```python
from build123d import *

# Parameters (mm, degrees)
F1_DEPTH = 63.5
F2_DEPTH = 25.4
F3_DEPTH = 7.9375
F0_W     = 21.7925966091
F0_H     = 28.575


with BuildPart() as f1:
    # F0 (on Front) → F1 (new body, symmetric)
    with BuildSketch(Plane.XZ):
        Polygon((31.6835418344, -20.7545107607), (-31.8164581656, -20.7545107607), (-31.8164581656, -39.8045107607), (50.7335418344, -39.8045107607), (50.7335418344, -20.7545107607), align=None)
    extrude(amount=F1_DEPTH, both=True)

    # F0 (on Front) → F2 (join, symmetric)
    with BuildSketch(Plane.XZ):
        with BuildLine():
            Line((31.6835418344, 16.0500892393), (31.6835418344, -20.7545107607))
            Line((31.6835418344, -20.7545107607), (50.7335418344, -20.7545107607))
            Line((50.7335418344, -20.7545107607), (50.7335418344, 16.0500892393))
            ThreePointArc((50.7335418344, 16.0500892393), (55.383221683, 27.2754093906), (66.6085418344, 31.9250892393))
            Line((66.6085418344, 31.9250892393), (77.2256346173, 31.9250892393))
            Line((77.2256346173, 31.9250892393), (77.2256346173, 50.9750892393))
            Line((77.2256346173, 50.9750892393), (66.6085418344, 50.9750892393))
            add(Edge.make_bspline(
                [(63.1497321777, 50.8033949922), (64.2990860037, 50.8698615177), (65.4521577964, 50.9270251755), (66.6085418344, 50.9750892393)],
                knots=[118.9365229564, 118.9365229564, 118.9365229564, 118.9365229564, 121.7892283462, 121.7892283462, 121.7892283462, 121.7892283462], degree=3))
            ThreePointArc((63.1497321777, 50.8033949922), (40.7188281216, 39.4910437606), (31.6835418344, 16.0500892393))
        make_face()
        Polygon((77.2256346173, 56.7154892393), (77.2256346173, 50.9750892393), (77.2256346173, 31.9250892393), (77.2256346173, 28.1404892393), (106.2330380082, 28.1404892393), (106.2330380082, 56.7154892393), align=None)
    extrude(amount=F2_DEPTH, both=True)

    # F0 (on Front) → F3 (join, symmetric)
    with BuildSketch(Plane.XZ):
        with BuildLine():
            add(Edge.make_bspline(
                [(-31.8164581656, -20.7545107607), (-26.2263988588, 29.0902056228), (15.2302560918, 48.0322369679), (63.1497321777, 50.8033949922)],
                knots=[0, 0, 0, 0, 118.9365229564, 118.9365229564, 118.9365229564, 118.9365229564], degree=3))
            Line((-31.8164581656, -20.7545107607), (31.6835418344, -20.7545107607))
            Line((31.6835418344, -20.7545107607), (31.6835418344, 16.0500892393))
            ThreePointArc((31.6835418344, 16.0500892393), (40.7188281216, 39.4910437606), (63.1497321777, 50.8033949922))
        make_face()
    extrude(amount=F3_DEPTH, both=True)

    # F0 (on Front) → F4 (revolve)
    with BuildSketch(Plane.XZ):
        with Locations((117.1293363128, 42.4279892393)):
            Rectangle(F0_W, F0_H)
    revolve(axis=Axis((106.2330380082, 0, 42.4279892393), (0, 0, -1)))


solid = f1.part
```
Source: CAD feature listing. Evaluate the final solid. Frame: model axes, mm. A direction names the side the tool comes from. Coordinates: 2 decimals unless noted, no trailing zeros. Loops run counter-clockwise (first coordinate to the right, second up) from the corner with the lowest first, then second, coordinate; pieces in that order, holes last. Notation, with made-up numbers: M 51.5,-33.75 L 63.5,-33.75 A21 cw 63.5,-29.75 Z; hole C 74.25,-20 d9. An arc over 180 degrees is marked long. Use CSV: the item, a comma, the result in double quotes.
(1) Cut plane A-A on z = -30.5. Return loops of the section in (x, y), and give its area (3 significant figures).
Answers follow:
outline,"M -31.82,-63.5 L 50.73,-63.5 L 50.73,63.5 L -31.82,63.5 Z"
area,"10,500 mm²"
(2) Reachability of faces 1 (the face through (31.684, 17, -2)), 2 (the face through (50.734, -1, -18)), 3 (the face through (72, 0, 31.925)), 4 (the face through (106.233, 24, 42)) from +Z, -Z, +X, -X, +Y, -Y: full face, straight path, thin tool, end or side. Return the list, or none.
Answers follow:
face 1,"+Z, -X, +Y"
face 2,"-Z, +X, +Y, -Y"
face 3,"-Z, +Y, -Y"
face 4,"+Z, -Z, +X, +Y"
(3) Line query: line 1 (Z direction, x = 96, y = -15.5); line 2 (Z direction, x = -14.5, y = -50.5); line 3 (X direction, y = -27.5, z = -21.5). Output: solid intervals per line, ascending. Write a range as [from, to].
Answers follow:
line 1,"[28.14, 56.72]"
line 2,"[-39.8, -20.75]"
line 3,"[-31.82, 50.73]"
(4) Contact query for flat-ended pins moving along their axis: pin 1 (3 mm diameter, centred on y = -2, z = 54.5, fed in from -X); pin 2 (1.1 mm diameter, centred on y = -4, z = 29, fed in from -X); pin 3 (1 mm diameter, centred on y = 6, z = -14, fed in from +X). Output: stop coordinate, or through.
Answers follow:
pin 1,"x = 77.23"
pin 2,"x = -5.98"
pin 3,"x = 50.73"
(5) Draft query along X for faces 5 (the face through (9, 63.5, -30)), 6 (the face through (31.684, -17, -2)), 7 (the face through (55.26, -0.36, 27.15)). Return one class per face: pulls with the +X half, pulls with the -X half, needs draft (parallel to the pull), parting line crosses it, or undercut.
Answers follow:
face 5,"needs draft"
face 6,"pulls with the -X half"
face 7,"undercut"
(6) Cut plane B-B on x = 97.5. Return loops of the section in (y, z), and give its area (3 significant figures).
Answers follow:
outline,"M -25.4,28.14 L 25.4,28.14 L 25.4,56.72 L -25.4,56.72 Z"
area,"1,450 mm²"
